Geometry: see drawing. Coordinates: mm, zero at the bounding-box minimum. A direction names the side the tool comes from. Coordinates: 2 decimals unless noted, no trailing zeros. Order: outer loops, then holes, each group sorted by start corner. A loop starts at its lowest first (then second) coordinate and runs counter-clockwise, first axis right, second up.
Item 1: Contact query for flat-ended pins moving along their axis: P1, Ø1.5, axis at y = 104.5, z = 31.5, coming from the -X side; P2, Ø4, axis at x = 162, y = 25.5, coming from the -Z side; P3, Ø1, axis at y = 23.5, z = 1, coming from the +X side; P4, Ø8, axis at x = 149, y = 114, coming from the +Z side. Output: stop coordinate, or through.
Item 2: Section D-D on y = 128. Return the cut outline in (x, z).
Item 3: Ray query, line 1 (X direction, y = 75, z = 14); line 2 (Y direction, x = 22.5, z = 37); line 3 (Z direction, x = 153, y = 22.5). Return the intervals inside material, ascending.
Item 4: Reachability of the marked faces 1, 2, 3, 4 and 5 from +Z, -Z, +X, -X, +Y, -Y: full face, straight path, thin tool, end or side. Return the list, or none.
Item 5: Section B-B on x = 26.5. Return the cut outline in (y, z), then the cut area to 3 significant figures.
Item 6: Section A-A on z = 27. Return the cut outline in (x, y).
Item 7: Section C-C on x = 162. Return the cut outline in (y, z).
Item 8: Mould query, pull axis Y, two halves, no side actions, for the marked faces 6, 7 and 8. Classes: released by +Y, released by -Y, zero draft, split by the parting line, or undercut.
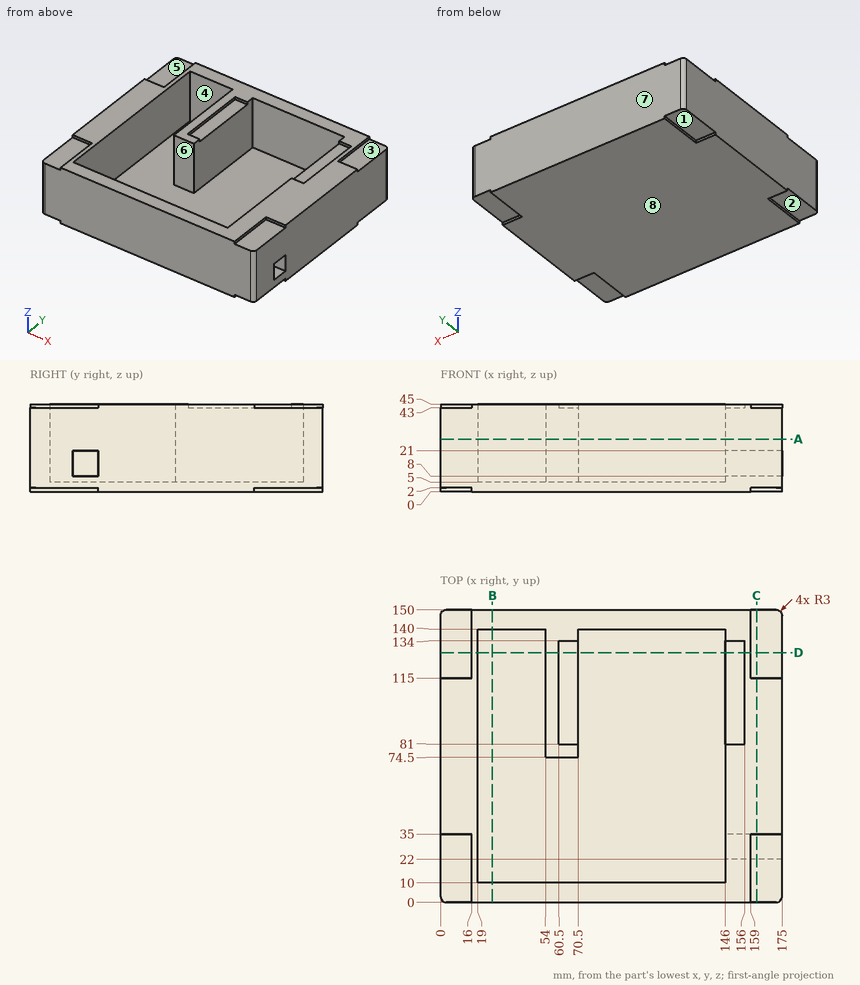
Answer list:
1. P1: stops at x = 0
1. P2: stops at z = 2
1. P3: stops at x = 159
1. P4: stops at z = 43
2. outline: (0, 2) - (16, 2) - (16, 0) - (159, 0) - (159, 2) - (175, 2) - (175, 43) - (159, 43) - (159, 45) - (156, 45) - (156, 43) - (146, 43) - (146, 5) - (70.5, 5) - (70.5, 43) - (60.5, 43) - (60.5, 45) - (54, 45) - (54, 5) - (19, 5) - (19, 45) - (16, 45) - (16, 43) - (0, 43) - close
3. line 1: x = 0 to 19, 54 to 70.5, 146 to 175
3. line 2: y = 0 to 10, 140 to 150
3. line 3: z = 0 to 8, 21 to 45
4. face 1: -Z, -X, +Y
4. face 2: -Z, -X, -Y
4. face 3: +Z, +X, +Y
4. face 4: +Z
4. face 5: +Z, -X, +Y
5. outline: (0, 0) - (150, 0) - (150, 45) - (140, 45) - (140, 5) - (10, 5) - (10, 45) - (0, 45) - close
5. area: 1,550 mm2
6. outline: (0, 3) arc R3 ccw to (3, 0) - (172, 0) arc R3 ccw to (175, 3) - (175, 147) arc R3 ccw to (172, 150) - (3, 150) arc R3 ccw to (0, 147) - close; hole (19, 10) - (146, 10) - (146, 140) - (70.5, 140) - (70.5, 74.5) - (54, 74.5) - (54, 140) - (19, 140) - close
7. outline: (0, 2) - (35, 2) - (35, 0) - (115, 0) - (115, 2) - (150, 2) - (150, 43) - (115, 43) - (115, 45) - (35, 45) - (35, 43) - (0, 43) - close; hole (22, 8) - (35, 8) - (35, 21) - (22, 21) - close
8. face 6: undercut
8. face 7: released by +Y
8. face 8: zero draft
